Input: part model. Units: mm. Frame: model coordinates. Round coordinates to 2 decimals unless told otherwise and drop trailing zeros. Loops run counter-clockwise (first coordinate to the right, second up) from the corner with the lowest first, then second, coordinate; pieces in that order, holes last. Notation, with made-up numbers: (-12.75, -13.75) -> (41.25, -13.75) arc R20 ccw to (41.25, 18.25) -> close; hole circle Ø10 at (68.25, 88). An arc over 180 degrees is marked (long way). One line per question, with ' | ' between items. Start each with the question number.
Q1. Contact query for flat-ended pins moving along their axis: P1, Ø1.5, axis at x = 1.5, z = 19.5, coming from the +Y side; P2, Ø1, axis at x = 1, y = -84, coming from the -Z side; P3, Ø0.9, axis at x = 1.5, y = -77.5, coming from the +Z side. Output: stop coordinate, or through.
Q2. Cut plane B-B on y = -76. Return loops of the section in (x, z), and give its area (3 significant figures).
Q3. Cut plane A-A on x = 0.55. Return loops of the section in (y, z).
Q4. Material intervals for L1, parallel to Y at x = 1.35, z = -3; L2, parallel to Y at x = 2.5, z = 18; L3, parallel to Z at x = 2.75, y = -59, sorted ascending.
from build123d import *

# Parameters (mm, degrees)
SKETCH_1_W          = 26
SKETCH_1_H          = 201
EXTRUDE_1_DEPTH     = 3
SKETCH_2_W          = 3
SKETCH_2_H          = 40
CUT_EXTRUDE_1_DEPTH = 3
FILLET_2_R          = 6
FILLET_3_R          = 6


with BuildPart() as part:
    # 草图1 → 凸台-拉伸1 (new body)
    with BuildSketch(Plane(origin=(0, 0, 0), x_dir=(0, 0, -1), z_dir=(1, 0, 0))):
        with Locations((-7.432605804, -18.101046442)):
            Rectangle(SKETCH_1_W, SKETCH_1_H)
    extrude(amount=EXTRUDE_1_DEPTH)

    # 草图2 → 切除-拉伸1 (cut)
    with BuildSketch(Plane(origin=(0, 0, 0), x_dir=(0, 0, -1), z_dir=(1, 0, 0))):
        with Locations((4.067394196, -68.601046442)):
            Rectangle(SKETCH_2_W, SKETCH_2_H)
        with Locations((-18.932605804, -68.601046442)):
            Rectangle(SKETCH_2_W, SKETCH_2_H)
        with Locations((-18.932605804, 32.398953558)):
            Rectangle(SKETCH_2_W, SKETCH_2_H)
        with Locations((4.067394196, 32.398953558)):
            Rectangle(SKETCH_2_W, SKETCH_2_H)
    extrude(amount=CUT_EXTRUDE_1_DEPTH, mode=Mode.SUBTRACT)

    # 圆角2
    fillet_2_edges = [part.edges().sort_by_distance(p)[0] for p in [
        (1.5, -118.601046442, 20.432605804),
    ]]
    fillet(fillet_2_edges, radius=FILLET_2_R)

    # 圆角3
    fillet_3_edges = [part.edges().sort_by_distance(p)[0] for p in [
        (1.5, 82.398953558, 20.432605804),
    ]]
    fillet(fillet_3_edges, radius=FILLET_3_R)


solid = part.part
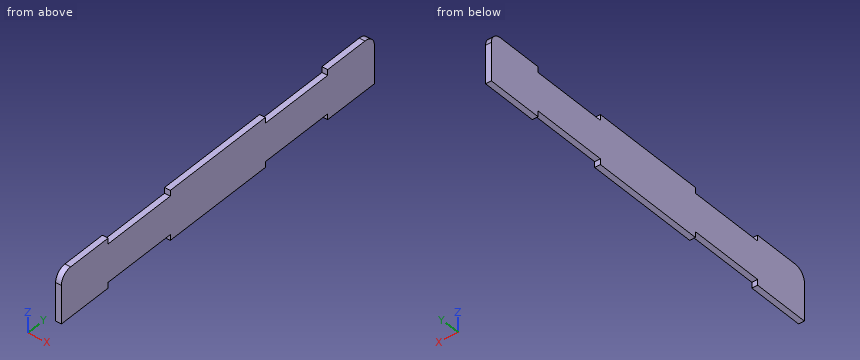
Results:
1) P1: y = 80.57 | P2: z = -2.57 | P3: z = 17.43
2) outline: (0, -2.57) -> (3, -2.57) -> (3, 17.43) -> (0, 17.43) -> close | area: 60.0 mm^2
3) outline: (-118.6, -5.57) -> (-88.6, -5.57) -> (-88.6, -2.57) -> (-48.6, -2.57) -> (-48.6, -5.57) -> (12.4, -5.57) -> (12.4, -2.57) -> (52.4, -2.57) -> (52.4, -5.57) -> (82.4, -5.57) -> (82.4, 14.43) arc R6 ccw to (76.4, 20.43) -> (52.4, 20.43) -> (52.4, 17.43) -> (12.4, 17.43) -> (12.4, 20.43) -> (-48.6, 20.43) -> (-48.6, 17.43) -> (-88.6, 17.43) -> (-88.6, 20.43) -> (-112.6, 20.43) arc R6 ccw to (-118.6, 14.43) -> close
4) L1: -118.6 to -88.6, -48.6 to 12.4, 52.4 to 82.4 | L2: -117.43 to -88.6, -48.6 to 12.4, 52.4 to 81.22 | L3: -2.57 to 17.43
